Geometry: final body of the model. Coordinates: model frame, mm. A direction names the side the tool comes from. Give positions to 0.01 mm unless a question says otherwise; leave off trailing zeros. Write each loop counter-clockwise with the first axis right and the second up, starting at its lowest first coordinate (ties: lowest second). Pieces come first, ordered by that corner, then holes.
```python
from build123d import *

# Parameters (mm, degrees)
CYLINDER043_R             = 3
CYLINDER043_DEPTH         = 10
CYLINDER042_R             = 3
CYLINDER042_DEPTH         = 10
CYLINDER041_R             = 3
CYLINDER041_DEPTH         = 10
CYLINDER044_R             = 3
CYLINDER044_DEPTH         = 10
CYLINDER019_R             = 3
CYLINDER019_DEPTH         = 12
CYLINDER018_R             = 25
CYLINDER018_DEPTH         = 12
BOX016_W                  = 70
BOX016_H                  = 50
BOX016_DEPTH              = 12
FUSION009_PLACEMENT_ANGLE = 90
BOX017_W                  = 10
BOX017_H                  = 100
BOX017_DEPTH              = 100
CYLINDER017_R             = 3
CYLINDER017_DEPTH         = 12
CYLINDER016_R             = 25
CYLINDER016_DEPTH         = 12
BOX015_W                  = 70
BOX015_H                  = 50
BOX015_DEPTH              = 12
FUSION008_PLACEMENT_ANGLE = 90


with BuildPart() as cilindro030:
    # Cylinder043 → Cylinder043 (new body)
    with BuildSketch(Plane(origin=(117, -31, 25), x_dir=(0, 0, 1), z_dir=(-1, 0, 0))):
        Circle(CYLINDER043_R)
    extrude(amount=CYLINDER043_DEPTH)


with BuildPart() as cilindro029:
    # Cylinder042 → Cylinder042 (new body)
    with BuildSketch(Plane(origin=(117, -111, 25), x_dir=(0, 0, 1), z_dir=(-1, 0, 0))):
        Circle(CYLINDER042_R)
    extrude(amount=CYLINDER042_DEPTH)


with BuildPart() as cilindro028:
    # Cylinder041 → Cylinder041 (new body)
    with BuildSketch(Plane(origin=(117, -31, 105), x_dir=(0, 0, 1), z_dir=(-1, 0, 0))):
        Circle(CYLINDER041_R)
    extrude(amount=CYLINDER041_DEPTH)


with BuildPart() as obj1:
    # Cylinder044 → Cylinder044 (new body)
    with BuildSketch(Plane(origin=(117, -111, 105), x_dir=(0, 0, 1), z_dir=(-1, 0, 0))):
        Circle(CYLINDER044_R)
    extrude(amount=CYLINDER044_DEPTH)

    # Fusion022: union Cilindro030, Cilindro029, Cilindro028
    add(cilindro030.part)
    add(cilindro029.part)
    add(cilindro028.part)


with BuildPart() as cilindro011:
    # Cylinder019 → Cylinder019 (new body)
    with BuildSketch(Plane(origin=(29, -45, -13), x_dir=(1, 0, 0), z_dir=(0, 0, 1))):
        Circle(CYLINDER019_R)
    extrude(amount=CYLINDER019_DEPTH)


with BuildPart() as cut018:
    # Cylinder018 → Cylinder018 (new body)
    with BuildSketch(Plane(origin=(29, -45, -13), x_dir=(1, 0, 0), z_dir=(0, 0, 1))):
        Circle(CYLINDER018_R)
    extrude(amount=CYLINDER018_DEPTH)

    # Cut018: cut Cilindro011
    add(cilindro011.part, mode=Mode.SUBTRACT)


with BuildPart() as lateral001:
    # Box016 → Box016 (new body)
    with BuildSketch(Plane(origin=(31, -70, -13), x_dir=(1, 0, 0), z_dir=(0, 0, 1))):
        with Locations((35, 25)):
            Rectangle(BOX016_W, BOX016_H)
    extrude(amount=BOX016_DEPTH)

    # Fusion009: union Cut018
    add(cut018.part)


with BuildPart() as lateral001_1:
    # Fusion009 placement: moved
    add(lateral001.part.moved(Location((16, -73, 105))).rotate(Axis((16, -73, 105), (1, 0, 0)), FUSION009_PLACEMENT_ANGLE))


with BuildPart() as obj2:
    # Box017 → Box017 (new body)
    with BuildSketch(Plane(origin=(107, -121, 15), x_dir=(1, 0, 0), z_dir=(0, 0, 1))):
        with Locations((5, 50)):
            Rectangle(BOX017_W, BOX017_H)
    extrude(amount=BOX017_DEPTH)


with BuildPart() as cilindro009:
    # Cylinder017 → Cylinder017 (new body)
    with BuildSketch(Plane(origin=(29, -45, -13), x_dir=(1, 0, 0), z_dir=(0, 0, 1))):
        Circle(CYLINDER017_R)
    extrude(amount=CYLINDER017_DEPTH)


with BuildPart() as cut017:
    # Cylinder016 → Cylinder016 (new body)
    with BuildSketch(Plane(origin=(29, -45, -13), x_dir=(1, 0, 0), z_dir=(0, 0, 1))):
        Circle(CYLINDER016_R)
    extrude(amount=CYLINDER016_DEPTH)

    # Cut017: cut Cilindro009
    add(cilindro009.part, mode=Mode.SUBTRACT)


with BuildPart() as cut038:
    # Box015 → Box015 (new body)
    with BuildSketch(Plane(origin=(31, -70, -13), x_dir=(1, 0, 0), z_dir=(0, 0, 1))):
        with Locations((35, 25)):
            Rectangle(BOX015_W, BOX015_H)
    extrude(amount=BOX015_DEPTH)

    # Fusion008: union Cut017
    add(cut017.part)


with BuildPart() as cut038_1:
    # Fusion008 placement: moved
    add(cut038.part.moved(Location((16, -34, 105))).rotate(Axis((16, -34, 105), (1, 0, 0)), FUSION008_PLACEMENT_ANGLE))

    # Fusion020: union lateral001, obj2
    add(lateral001_1.part)
    add(obj2.part)

    # Cut038: cut obj1
    add(obj1.part, mode=Mode.SUBTRACT)


solid = cut038_1.part
```
Item 1: Pull-direction query (Y, two-part tool) for faces 6 (the face through (112.1, -112.8, 22.6)), 7 (the face through (112, -31, 22)), 8 (the face through (47, -27, 60)), 9 (the face through (112, -121, 64)); classes: +Y half, -Y half, draft (parallel to the pull), parting line (faces both ways), or undercut.
Found:
face 6: undercut
face 7: undercut
face 8: draft
face 9: -Y half
Item 2: Section B-B, the plane z = 105. Return the cut outline in (x, y).
Found:
outline: (107, -121) - (117, -121) - (117, -114) - (107, -114) - close; (107, -108) - (117, -108) - (117, -34) - (107, -34) - close; (107, -28) - (117, -28) - (117, -21) - (107, -21) - close
Item 3: Section A-A, the plane y = -31. Return the cut outline in (x, z).
Found:
outline: (47, 35) - (107, 35) - (107, 28) - (117, 28) - (117, 102) - (107, 102) - (107, 85) - (47, 85) - (47, 84.92) arc R25 ccw (long way) to (47, 35.08) - close; (107, 15) - (117, 15) - (117, 22) - (107, 22) - close; (107, 108) - (117, 108) - (117, 115) - (107, 115) - close; hole (47, 57.76) - (47, 62.24) arc R3 ccw (long way) to start
Item 4: Line query: L1, parallel to Y at x = 114.5, z = 105; L2, parallel to Y at x = 31, z = 57.5; L3, parallel to Z at x = 45, y = -62.75. Output: solid intervals per line, ascending.
Found:
L1: y = -121 to -114, -108 to -34, -28 to -21
L2: y = -72 to -60, -33 to -21
L3: z = 35 to 57, 63 to 85
Item 5: Reachability of faces 1 (the face through (77, -27, 85)), 2 (the face through (47, -66, 60)), 3 (the face through (77, -66, 35)), 4 (the face through (63, -72, 60)), 5 (the face through (63, -33, 60)) from +Z, -Z, +X, -X, +Y, -Y: full face, straight path, thin tool, end or side. Return the list, or none.
Found:
face 1: +Z, -X, +Y, -Y
face 2: +Y, -Y
face 3: -Z, -X, +Y, -Y
face 4: +Z, -Z, -X, -Y
face 5: +Z, -Z, -X
Item 6: Section D-D, the plane x = 84. Return the cut outline in (y, z).
Found:
outline: (-72, 35) - (-60, 35) - (-60, 85) - (-72, 85) - close; (-33, 35) - (-21, 35) - (-21, 85) - (-33, 85) - close
Item 7: Pin query (flat end, axial travel): pin 1 Ø13 at (x, y) = (64.5, -68) entering from +Z; pin 2 Ø5 at (y, z) = (-111, 25) entering from -X; pin 3 Ø3.5 at (x, y) = (68, -28) entering from -Z; pin 4 Ø9.5 at (x, z) = (45, 60) entering from -Y. Return the tip coordinate at first contact, or that it passes through.
Found:
pin 1: stops at z = 85
pin 2: passes through
pin 3: stops at z = 35
pin 4: stops at y = -72
Item 8: Section C-C, the plane x = 45. Return the cut outline in (y, z), plus the area to 3 significant figures.
Found:
outline: (-72, 35) - (-60, 35) - (-60, 57) - (-72, 57) - close; (-72, 63) - (-60, 63) - (-60, 85) - (-72, 85) - close; (-33, 35) - (-21, 35) - (-21, 57) - (-33, 57) - close; (-33, 63) - (-21, 63) - (-21, 85) - (-33, 85) - close
area: 1,060 mm2
